Autodesk Inventor part; units mm, degrees
ref_plane "YZ Plane" through (0, 0, 0) normal (1, 0, 0) x (0, 1, 0)
ref_plane "XZ Plane" through (0, 0, 0) normal (0, 1, 0) x (-1, 0, 0)
ref_plane "XY Plane" through (0, 0, 0) normal (0, 0, 1) x (1, 0, 0)
sketch "Sketch1" plane through (0, 0, 0) normal (0, 1, 0) x (-1, 0, 0)
  line L0 (0, 0) -> (0, -53)
  circle A0 centre (0, 0) radius 4
  circle A1 centre (0, -53) radius 4
  line L1 (0, 10) -> (10, 10)
  line L2 (0, -63) -> (-10, -63)
  line L3 (10, 10) -> (-10, 10)
  line L4 (-10, 10) -> (-10, -63)
  line L5 (-10, -63) -> (10, -63)
  line L6 (10, -63) -> (10, 10)
  dimension "d0" = 53
  dimension "d1" = 8
  dimension "d2" = 8
  dimension "d3" = 10
  dimension "d4" = 10
  dimension "d5" = 10
  dimension "d6" = 10
  dimension "d8" = 10
  dimension "d9" = 10
  dimension "d10" = 73
extrude "Extrusion1" add sketch "Sketch1" along normal blind 54
fillet "Fillet1" radius 2 4 edges at (10, 27, 10) (-10, 27, 10) (10, 27, -63) (-10, 27, -63)
properties part number "Bearing Seats"
The model under review builds one solid part; all positions refer to its coordinate system, in mm. Coordinates: 2 decimals unless noted, no trailing zeros. Write each loop counter-clockwise with the first axis right and the second up, starting at its lowest first coordinate (ties: lowest second). Pieces come first, ordered by that corner, then holes. Notation, with made-up numbers: (59.5, -2.5) -> (96.5, -2.5) arc R22 ccw to (96.5, 29.5) -> close; hole circle Ø7 at (-27.75, 80). An arc over 180 degrees is marked (long way). One line per item, written item: value. Start each with the question number.
Q1. Clearance check with a flat-ended pin moving along its axis: P1, Ø6.5, axis at x = 0, z = -53, coming from the -Y side (3 decimals). State where the tip first meets the part, or that it passes through.
Q2. Add section B-B, the plane x = 0. Give the boundary of the cut face in (y, z).
Q3. To check wall thickness, follow probe 1 along Z at (x, y) = (0, 24); probe 2 along X at (y, z) = (31.5, 0); probe 3 along Z at (x, y) = (-1.5, 46.5). State the ranges of each line that lie inside material, in increasing order.
Q4. Add section A-A, the plane z = -53. Give the boundary of the cut face in (x, y).
Q5. Add section C-C, the plane y = 7.5. Give the boundary of the cut face in (x, z), then the cut area to 3 significant figures.
Q6. The part is to be moulded in two halves that separate along X. For faces 1 (the face through (9.4, 27.38, 9.43)), 2 (the face through (0.867, 26.622, 3.905)), 3 (the face through (0, 0, -26)), 4 (the face through (0.867, 26.622, -49.095)), say which applies: +X half, -X half, draft (parallel to the pull), parting line (faces both ways), or undercut.
Response:
1. P1: through
2. outline: (0, -63) -> (54, -63) -> (54, -57) -> (0, -57) -> close; (0, -49) -> (54, -49) -> (54, -4) -> (0, -4) -> close; (0, 4) -> (54, 4) -> (54, 10) -> (0, 10) -> close
3. probe 1: -63 to -57, -49 to -4, 4 to 10
3. probe 2: -10 to -4, 4 to 10
3. probe 3: -63 to -56.71, -49.29 to -3.71, 3.71 to 10
4. outline: (-10, 0) -> (-4, 0) -> (-4, 54) -> (-10, 54) -> close; (4, 0) -> (10, 0) -> (10, 54) -> (4, 54) -> close
5. outline: (-10, -61) arc R2 ccw to (-8, -63) -> (8, -63) arc R2 ccw to (10, -61) -> (10, 8) arc R2 ccw to (8, 10) -> (-8, 10) arc R2 ccw to (-10, 8) -> close; hole circle Ø8 at (0, -53); hole circle Ø8 at (0, 0)
5. area: 1,360 mm²
6. face 1: +X half
6. face 2: undercut
6. face 3: draft
6. face 4: undercut
